Source: three-view drawing plus pictorial views. Frame: mm from the lowest corner of the part. A direction names the side the tool comes from. Give positions to 0.01 mm unless a question says otherwise; leave off trailing zeros. Order: outer loops, then holes, each group sorted by start corner. A loop starts at its lowest first (then second) coordinate and runs counter-clockwise, first axis right, second up. Notation, with made-up numbers: (9.25, -29.75) -> (35.25, -29.75) arc R26 cw to (35.25, -0.75) -> close; hole circle Ø4 at (-17.5, 49.5). An arc over 180 degrees is marked (long way). Write item = value, one per line.
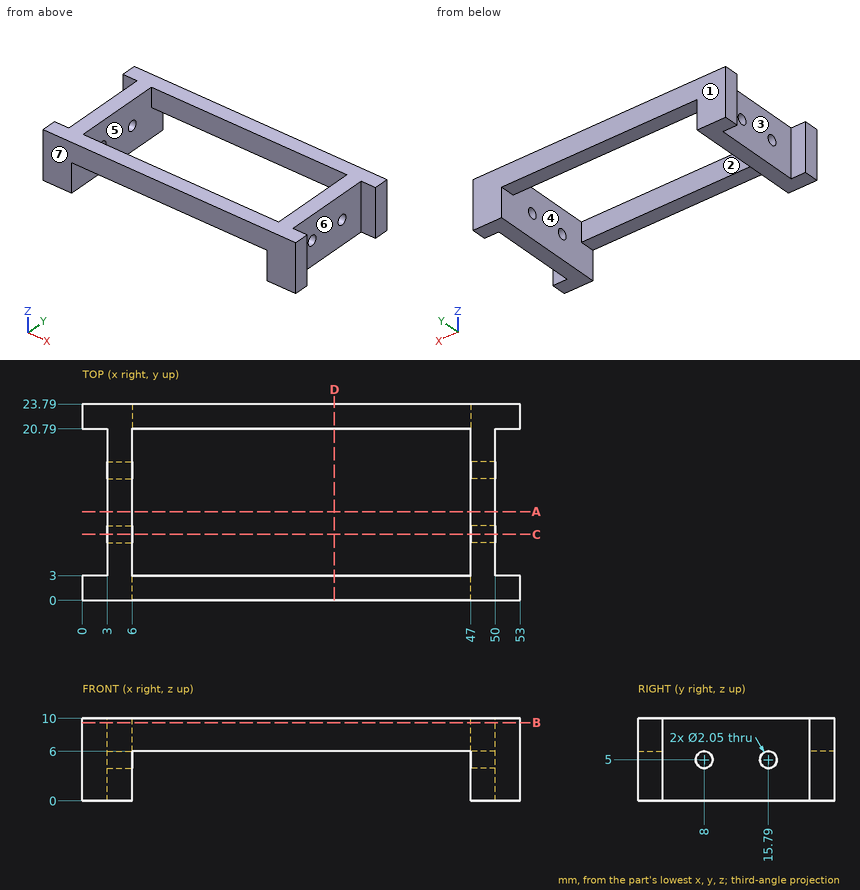
1) Mould query, pull axis X, two halves, no side actions, for the marked faces 5, 6 and 7. Classes: +X half, -X half, draft (parallel to the pull), parting line (faces both ways), or undercut.
Check sheet entries:
face_5 = undercut
face_6 = +X half
face_7 = draft
2) Section query D-D (x = 30.5). Output: boundary loops of the cut face in (y, z).
Check sheet entries:
outline = (0, 6) -> (3, 6) -> (3, 10) -> (0, 10) -> close; (20.79, 6) -> (23.79, 6) -> (23.79, 10) -> (20.79, 10) -> close
3) Section query A-A (y = 10.75). Output: boundary loops of the cut face in (x, z), plus the area to 3 significant figures.
Check sheet entries:
outline = (3, 0) -> (6, 0) -> (6, 10) -> (3, 10) -> close; (47, 0) -> (50, 0) -> (50, 10) -> (47, 10) -> close
area = 60.0 mm²
4) First-contact query: P1, Ø2, axis at y = 4.5, z = 7, coming from the +X side; P2, Ø1.6, axis at y = 15.79, z = 5, coming from the -X side; P3, Ø3, axis at x = 13, y = 3, coming from the -Z side; P4, Ø3, axis at y = 7, z = 4.5, coming from the -X side. Flat tips, straight axial feed; report the tip coordinate or a pass-through.
Check sheet entries:
P1 = 50
P2 = through
P3 = 6
P4 = 3
5) Section query C-C (y = 8). Output: boundary loops of the cut face in (x, z) (3 decimals).
Check sheet entries:
outline = (3, 0) -> (6, 0) -> (6, 3.975) -> (3, 3.975) -> close; (3, 6.025) -> (6, 6.025) -> (6, 10) -> (3, 10) -> close; (47, 0) -> (50, 0) -> (50, 3.975) -> (47, 3.975) -> close; (47, 6.025) -> (50, 6.025) -> (50, 10) -> (47, 10) -> close
6) Section query B-B (z = 9.5). Output: boundary loops of the cut face in (x, y).
Check sheet entries:
outline = (0, 0) -> (53, 0) -> (53, 3) -> (50, 3) -> (50, 20.79) -> (53, 20.79) -> (53, 23.79) -> (0, 23.79) -> (0, 20.79) -> (3, 20.79) -> (3, 3) -> (0, 3) -> close; hole (6, 3) -> (47, 3) -> (47, 20.79) -> (6, 20.79) -> close
7) Line query: line 1 (Y direction, x = 5.25, z = 5) (3 decimals); line 2 (X direction, y = 7, z = 4.5); line 3 (X direction, y = 2.75, z = 5.75). Output: solid intervals per line, ascending. Write a range as from..to.
Check sheet entries:
line_1 = 0..6.975, 9.025..14.765, 16.815..23.79
line_2 = 3..6, 47..50
line_3 = 0..6, 47..53
8) Reachability of the marked faces 1, 2, 3 and 4 from +Z, -Z, +X, -X, +Y, -Y: full face, straight path, thin tool, end or side. Return the list, or none.
Check sheet entries:
face_1 = +Z, -Z, +X, -X, +Y
face_2 = +Z, -Z
face_3 = +Z, -Z, -X
face_4 = -Z
